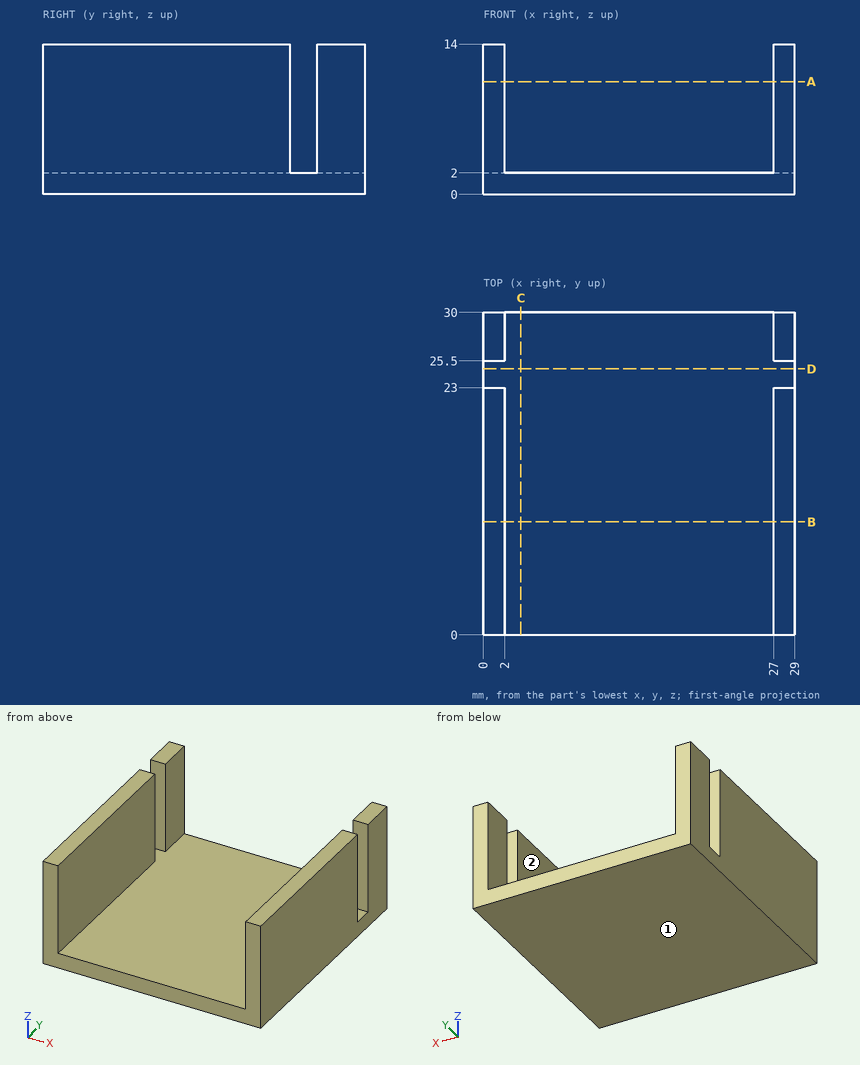
Verification items for this drawing (mm, ordinates from the low corner). A direction names the side the tool comes from. Coordinates: 2 decimals unless noted, no trailing zeros. Loops run counter-clockwise (first coordinate to the right, second up) from the corner with the lowest first, then second, coordinate; pieces in that order, holes last. Notation, with made-up numbers: (33, -33) -> (46, -33) arc R24 cw to (46, -10) -> close; hole circle Ø4 at (5, 64). An arc over 180 degrees is marked (long way). Answer in a Markdown table with one row per item. Add a question column.
1. Section check A-A, the plane z = 10.5. Enter the section's corners in (x, y).
2. Section check B-B, the plane y = 10.5. Enter the section's corners in (x, z), then the cut area to 3 significant figures.
3. Depth check by flat-ended pin: P1, Ø6, axis at x = 18.5, y = 18.5, coming from the +Z side. Enter the tip coordinate at first touch or a pass-through.
4. Section check D-D, the plane y = 24.75. Enter the section's corners in (x, z), then the cut area to 3 significant figures.
5. Material ranges on probe 1 along X at (y, z) = (22.5, 7.75); probe 2 along Z at (x, y) = (4.25, 20.25), recorded low to high. Write a range as [from, to].
6. Section check C-C, the plane x = 3.5. Enter the section's corners in (y, z), then the cut area to 3 significant figures.
7. Access from +Z, -Z, +X, -X, +Y, -Y to the whole of each face (thin tool, end or side, straight path). Record for the marked faces 1 and 2.
Derived:
| question | item | result |
|---|---|---|
| 1 | outline | (0, 0) -> (2, 0) -> (2, 23) -> (0, 23) -> close; (0, 25.5) -> (2, 25.5) -> (2, 30) -> (0, 30) -> close; (27, 0) -> (29, 0) -> (29, 23) -> (27, 23) -> close; (27, 25.5) -> (29, 25.5) -> (29, 30) -> (27, 30) -> close |
| 2 | outline | (0, 0) -> (29, 0) -> (29, 14) -> (27, 14) -> (27, 2) -> (2, 2) -> (2, 14) -> (0, 14) -> close |
| 2 | area | 106 mm² |
| 3 | P1 | stops at z = 2 |
| 4 | outline | (0, 0) -> (29, 0) -> (29, 2) -> (0, 2) -> close |
| 4 | area | 58.0 mm² |
| 5 | probe 1 | x = [0, 2], [27, 29] |
| 5 | probe 2 | z = [0, 2] |
| 6 | outline | (0, 0) -> (30, 0) -> (30, 2) -> (0, 2) -> close |
| 6 | area | 60.0 mm² |
| 7 | face 1 | -Z, +X, -X, +Y, -Y |
| 7 | face 2 | +Z, +Y, -Y |
